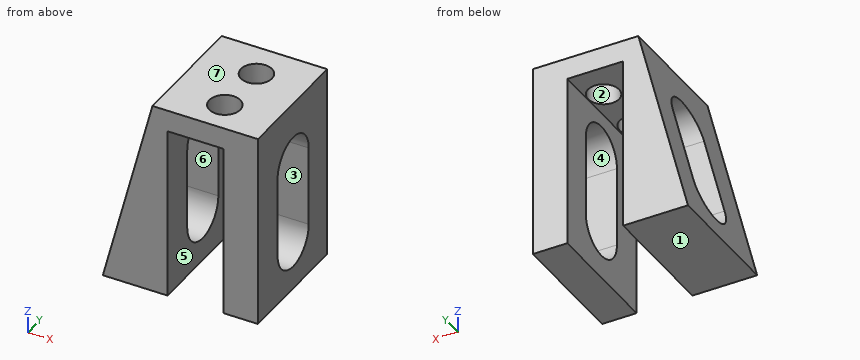
from build123d import *

# Parameters (mm, degrees)
F1_DEPTH = 20
F2_R     = 2.5
F3_DEPTH = 10
F5_W     = 9
F5_H     = 28
F6_DEPTH = 25
F7_W     = 9
F7_H     = 13
F8_DEPTH = 25


with BuildPart() as f1:
    # F0 (on Front) → F1 (new body)
    with BuildSketch(Plane.XZ):
        Polygon((-49.089543, 31.5), (-57.089543, 0), (-32.089543, 0), (-32.089543, 31.5), align=None)
    extrude(amount=F1_DEPTH)

    # F2 (on face) → F3 (cut)
    with BuildSketch(Plane.XY.offset(31.5)):
        with Locations((-40.230012, -5.844655)):
            Circle(F2_R)
        with Locations((-40.32638, -14.806874)):
            Circle(F2_R)
    extrude(amount=-F3_DEPTH, mode=Mode.SUBTRACT)

    # F5 (on face) → F6 (cut)
    with BuildSketch(Plane.XZ.offset(20)):
        with Locations((-42.152388, 14)):
            Rectangle(F5_W, F5_H)
    extrude(amount=-F6_DEPTH, mode=Mode.SUBTRACT)

    # F7 (on face) → F8 (cut)
    with BuildSketch(Plane.YZ.offset(-32.089543)):
        with BuildLine():
            ThreePointArc((-5.334587, 21.249529), (-9.834587, 25.749529), (-14.334587, 21.249529))
            Line((-14.334587, 21.249529), (-5.334587, 21.249529))
        make_face()
        with Locations((-9.834587, 14.749529)):
            Rectangle(F7_W, F7_H)
        with BuildLine():
            Line((-5.334587, 8.249529), (-14.334587, 8.249529))
            ThreePointArc((-14.334587, 8.249529), (-9.834587, 3.749529), (-5.334587, 8.249529))
        make_face()
    extrude(amount=-F8_DEPTH, mode=Mode.SUBTRACT)


solid = f1.part
Work out the finished part from the listing and answer in its coordinate system (mm). Face numbers are marked on the shaded views. A direction names the side the tool comes from. Round coordinates to 2 decimals unless told otherwise and drop trailing zeros. Write each loop counter-clockwise with the first axis right and the second up, starting at its lowest first coordinate (ties: lowest second). Pieces come first, ordered by that corner, then holes. Notation, with made-up numbers: (-37.5, 38) - (-27.5, 38) arc R13 ccw to (-27.5, 55) - close; hole circle Ø9 at (18.25, -16.75). An arc over 180 degrees is marked (long way). Answer in a Markdown table with one row per item. Add a question column.
1. Find the intervals of material crossed by line 1 along Y through (x, z) = (-51, 21); line 2 along Z through (x, y) = (-45, -9.5); line 3 along X through (y, z) = (-18.5, 24), in increasing order. Write a range as from..to.
2. For the marked faces 5, 6 and 7, determine the directions among +Z, -Z, +X, -X, +Y, -Y from which every point of the face is accessible in a straight line to the end or side of a thin tool.
3. The mould has two halves that part along Z. Classify the marked faces 1, 2, 3 and 4: +Z half, -Z half, draft (parallel to the pull), parting line (faces both ways), or undercut.
4. Given pin 1 (8 mm diameter, centred on y = -13.5, z = 10, fed in from -X); pin 2 (2 mm diameter, centred on y = -9, z = 4, fed in from -X); pin 3 (2.5 mm diameter, centred on x = -40, y = -11.5, fed in from -Z), each flat-ended and moving along its own axis, determine where each tip first touches the part or whether it passes through.
5. A cutting plane is placed at C-C, the plane x = -39. Determine the outline of the cut face in (y, z), and give its area (3 significant figures).
6. A cutting plane is placed at D-D, the plane y = -7. Determine the outline of the cut face in (x, z), and give its area (3 significant figures).
7. A cutting plane is placed at A-A, the plane y = -19. Determine the outline of the cut face in (x, z), and give its area (4 significant figures).
8. A cutting plane is placed at B-B, the plane z = 17.5. Determine the outline of the cut face in (x, y).
Worked out:
| question | item | result |
|---|---|---|
| 1 | line 1 | -20..-14.33, -5.33..0 |
| 1 | line 2 | 28..31.5 |
| 1 | line 3 | -50.99..-46.65, -37.65..-32.09 |
| 2 | face 5 | -Z, +Y, -Y |
| 2 | face 6 | +X, -X |
| 2 | face 7 | +Z, +X, -X, +Y, -Y |
| 3 | face 1 | -Z half |
| 3 | face 2 | draft |
| 3 | face 3 | undercut |
| 3 | face 4 | undercut |
| 4 | pin 1 | x = -55.56 |
| 4 | pin 2 | x = -56.33 |
| 4 | pin 3 | z = 28 |
| 5 | outline | (-20, 28) - (-16.93, 28) - (-16.93, 31.5) - (-20, 31.5) - close; (-12.69, 28) - (-8.02, 28) - (-8.02, 31.5) - (-12.69, 31.5) - close; (-3.67, 28) - (0, 28) - (0, 31.5) - (-3.67, 31.5) - close |
| 5 | area | 39.9 mm^2 |
| 6 | outline | (-57.09, 0) - (-46.65, 0) - (-46.65, 4.75) - (-55.88, 4.75) - close; (-50.81, 24.74) - (-46.65, 24.74) - (-46.65, 28) - (-42.45, 28) - (-42.45, 31.5) - (-49.09, 31.5) - close; (-38.01, 28) - (-37.65, 28) - (-37.65, 24.74) - (-32.09, 24.74) - (-32.09, 31.5) - (-38.01, 31.5) - close; (-37.65, 0) - (-32.09, 0) - (-32.09, 4.75) - (-37.65, 4.75) - close |
| 6 | area | 149 mm^2 |
| 7 | outline | (-57.09, 0) - (-46.65, 0) - (-46.65, 28) - (-37.65, 28) - (-37.65, 0) - (-32.09, 0) - (-32.09, 31.5) - (-49.09, 31.5) - close |
| 7 | area | 409.5 mm^2 |
| 8 | outline | (-52.65, -20) - (-46.65, -20) - (-46.65, -14.33) - (-52.65, -14.33) - close; (-52.65, -5.33) - (-46.65, -5.33) - (-46.65, 0) - (-52.65, 0) - close; (-37.65, -20) - (-32.09, -20) - (-32.09, -14.33) - (-37.65, -14.33) - close; (-37.65, -5.33) - (-32.09, -5.33) - (-32.09, 0) - (-37.65, 0) - close |
